from build123d import *

# Parameters (mm, degrees)
F0_W     = 36.8
F0_H     = 1.5
F0_W_2   = 1.5
F1_DEPTH = 25
F2_DEPTH = 100
F0_H_2   = 10.5
F3_DEPTH = 2
F4_R     = 3
F5_W     = 36.8
F5_H     = 16.8
F6_DEPTH = 2


with BuildPart() as f1:
    # F0 (on Top) → F1 (new body)
    with BuildSketch(Plane.XY):
        with Locations((19.9, 19.05)):
            Rectangle(F0_W, F0_H)
        with Locations((39.05, 19.05)):
            Rectangle(F0_W_2, F0_H)
        Polygon((0, 18.3), (0, 0), (39.8, 0), (39.8, 18.3), (38.3, 18.3), (38.3, 1.5), (1.5, 1.5), (1.5, 18.3), align=None)
        with Locations((0.75, 19.05)):
            Rectangle(F0_W_2, F0_H)
    extrude(amount=F1_DEPTH)

    # F0 (on Top) → F2 (join)
    with BuildSketch(Plane.XY):
        Polygon((0, 31.8), (0, 19.8), (1.5, 19.8), (1.5, 30.3), (38.3, 30.3), (38.3, 19.8), (39.8, 19.8), (39.8, 31.8), align=None)
        Polygon((0, 18.3), (0, 0), (39.8, 0), (39.8, 18.3), (38.3, 18.3), (38.3, 1.5), (1.5, 1.5), (1.5, 18.3), align=None)
        with Locations((39.05, 19.05)):
            Rectangle(F0_W_2, F0_H)
        with Locations((0.75, 19.05)):
            Rectangle(F0_W_2, F0_H)
    extrude(amount=-F2_DEPTH)

    # F0 (on Top) → F3 (join)
    with BuildSketch(Plane.XY):
        with Locations((19.9, 25.05)):
            Rectangle(F0_W, F0_H_2)
        with Locations((19.9, 19.05)):
            Rectangle(F0_W, F0_H)
    extrude(amount=-F3_DEPTH)

    # F4
    f4_edges = [f1.edges().sort_by_distance(p)[0] for p in [
        (19.9, 18.3, -2),
    ]]
    fillet(f4_edges, radius=F4_R)

    # F5 (on face) → F6 (join)
    with BuildSketch(Plane.XY.offset(25)):
        with Locations((19.9, 9.9)):
            Rectangle(F5_W, F5_H)
    extrude(amount=-F6_DEPTH)


solid = f1.part
Can you work these out from the model? Positions are in its coordinate system, mm. A direction names the side the tool comes from. Round coordinates to 2 decimals unless told otherwise and drop trailing zeros. Order: outer loops, then holes, each group sorted by start corner. A loop starts at its lowest first (then second) coordinate and runs counter-clockwise, first axis right, second up. Notation, with made-up numbers: (68, 56.25) -> (121, 56.25) arc R15 ccw to (121, 66.25) -> close; hole circle Ø4 at (0.5, 7.5). An arc over 180 degrees is marked (long way). Write each question's results on one line, items separated by ' | '. Start each with the question number.
Item 1: Please list where these lines run through material, in increasing order: L1, parallel to X at y = 11, z = -7; L2, parallel to Y at x = 6, z = -19; L3, parallel to Y at x = 20, z = 6.
Item 2: Thinking about a two-plate mould opening in X: for faces 1 (the flat face through (0, 16, -37)), 2 (the flat face through (38.3, 16, -38)), 3 (the flat face through (20, 31.8, -49)), 4 (the flat face through (1.5, 16, -38)), which applies, +X half, -X half, draft (parallel to the pull), parting line (faces both ways), or undercut?
Item 3: If we section it at B-B, the plane x = 22: Write out the boundary of the cut face in (y, z).
Item 4: Will these pins go through, and if not, where does the flat tip stop? pin 1 (8.5 mm diameter, centred on x = 28.5, y = 7.5, fed in from -Z); pin 2 (20 mm diameter, centred on x = 29.5, z = 15.5, fed in from +Y); pin 3 (3 mm diameter, centred on x = 22.5, y = 22.5, fed in from -Z).
Item 5: If we section it at D-D, the plane z = 14.5: Write out the boundary of the cut face in (x, y).
Item 6: If we section it at C-C, the plane y = 4.5: Write out the boundary of the cut face in (x, z).
Item 7: Which directions (+Z, -Z, +X, -X, +Y, -Y) give clear straight access to the entire face, cutting with the end or side of a thin tool? Please do faces 5 (the flat face through (20, 0, -37)), 6 (the flat face through (20, 10, 23)), 7 (the flat face through (20, 26, 0)).
Item 8: If we section it at A-A, the plane z = -51: Write out the boundary of the cut face in (x, y), then the cut area to 3 significant figures.
Results:
1) L1: x = 0 to 1.5, 38.3 to 39.8 | L2: y = 0 to 1.5, 30.3 to 31.8 | L3: y = 0 to 1.5, 18.3 to 19.8
2) face 1: -X half | face 2: undercut | face 3: draft | face 4: undercut
3) outline: (0, -100) -> (1.5, -100) -> (1.5, 23) -> (18.3, 23) -> (18.3, 1) arc R3 ccw to (21.3, -2) -> (30.3, -2) -> (30.3, -100) -> (31.8, -100) -> (31.8, 0) -> (19.8, 0) -> (19.8, 25) -> (0, 25) -> close
4) pin 1: stops at z = 23 | pin 2: stops at y = 19.8 | pin 3: stops at z = -2
5) outline: (0, 0) -> (39.8, 0) -> (39.8, 19.8) -> (0, 19.8) -> close; hole (1.5, 1.5) -> (38.3, 1.5) -> (38.3, 18.3) -> (1.5, 18.3) -> close
6) outline: (0, -100) -> (1.5, -100) -> (1.5, 23) -> (38.3, 23) -> (38.3, -100) -> (39.8, -100) -> (39.8, 25) -> (0, 25) -> close
7) face 5: +Z, -Z, +X, -X, -Y | face 6: -Z | face 7: +Z, +X, -X, +Y
8) outline: (0, 0) -> (39.8, 0) -> (39.8, 31.8) -> (0, 31.8) -> close; hole (1.5, 1.5) -> (38.3, 1.5) -> (38.3, 30.3) -> (1.5, 30.3) -> close | area: 206 mm2
